```python
from build123d import *

# Parameters (mm, degrees)
F0_R     = 10
F1_DEPTH = 40
F3_D     = 10


# Not quite as in the source:
# - a feature names something its author has since deleted; it is built from what else it names


with BuildPart() as f1:
    # F0 (on Front) → F1 (new body)
    with BuildSketch(Plane.XZ):
        with BuildLine():
            ThreePointArc((-24.4948974278, 0), (-21.3326197677, -1.1270166538), (-19.5959179423, -4))
            ThreePointArc((-19.5959179423, -4), (0, -20), (19.5959179423, -4))
            ThreePointArc((19.5959179423, -4), (21.3326197677, -1.1270166538), (24.4948974278, 0))
            Line((24.4948974278, 0), (35, 0))
            ThreePointArc((35, 0), (38.5355339059, 1.4644660941), (40, 5))
            Line((40, 5), (40, 20))
            Line((40, 20), (-40, 20))
            Line((-40, 20), (-40, 5.3399834782))
            ThreePointArc((-40, 5.3399834782), (-38.6653317972, 1.5867843161), (-35.0115722683, 0))
            Line((-35.0115722683, 0), (-24.4948974278, 0))
        make_face()
        Circle(F0_R, mode=Mode.SUBTRACT)
    extrude(amount=F1_DEPTH)

    # F3 (through all)
    with Locations(Plane.XY.offset(20)):
        with Locations((-30, -10), (-29.9999981744, -30), (30, -30), (30, -10)):
            Hole(F3_D / 2)


solid = f1.part
```
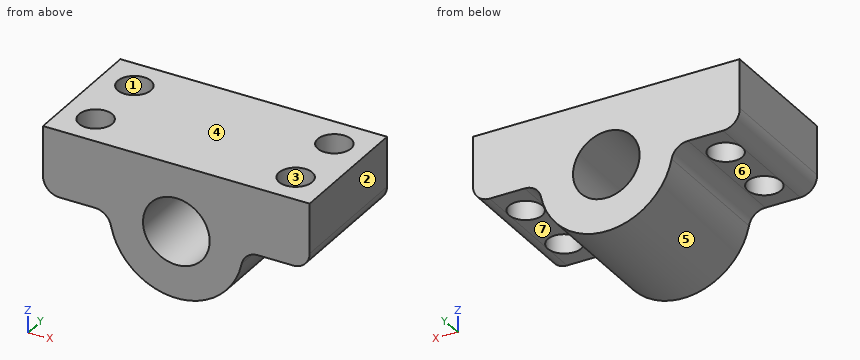
Here's how the part is built. I have some questions about the finished solid (model axes, mm). Face numbers are marked on the shaded views. A direction names the side the tool comes from. Give positions to 0.01 mm unless a question says otherwise; leave off trailing zeros. Write each loop counter-clockwise with the first axis right and the second up, starting at its lowest first coordinate (ties: lowest second). Pieces come first, ordered by that corner, then holes.
(1) Imagine slicing it at C-C, the plane z = 4. Write out the boundary of the cut face in (x, y).
Output values:
outline: (-39.91, -40) - (-9.17, -40) - (-9.17, 0) - (-39.91, 0) - close; (9.17, -40) - (39.9, -40) - (39.9, 0) - (9.17, 0) - close; hole circle Ø10 at (-30, -30); hole circle Ø10 at (-30, -10); hole circle Ø10 at (30, -30); hole circle Ø10 at (30, -10)
(2) Imagine slicing it at B-B, the plane x = -30. Write out the boundary of the cut face in (y, z).
Output values:
outline: (-40, 0) - (-35, 0) - (-35, 20) - (-40, 20) - close; (-25, 0) - (-15, 0) - (-15, 20) - (-25, 20) - close; (-5, 0) - (0, 0) - (0, 20) - (-5, 20) - close
(3) Thinking about a two-plate mould opening in X: for the marked faces 1, 2, 3 and 4, which applies, pulls with the +X half, pulls with the -X half, needs draft (parallel to the pull), parting line crosses it, or undercut?
Output values:
face 1: undercut
face 2: pulls with the +X half
face 3: undercut
face 4: needs draft
(4) Imagine slicing it at A-A, the plane y = -33. Write out the boundary of the cut face in (x, z), and give its area (3 significant figures).
Output values:
outline: (-40, 5.34) arc R5 ccw to (-35.01, 0) - (-34, 0) - (-34, 20) - (-40, 20) - close; (-26, 0) - (-24.49, 0) arc R5 cw to (-19.6, -4) arc R20 ccw to (19.6, -4) arc R5 cw to (24.49, 0) - (26, 0) - (26, 20) - (-26, 20) - close; (34, 0) - (35, 0) arc R5 ccw to (40, 5) - (40, 20) - (34, 20) - close; hole circle Ø20 at (0, 0)
area: 1,590 mm2
(5) Imagine slicing it at D-D, the plane x = 0. Write out the boundary of the cut face in (y, z), and give its area (3 significant figures).
Output values:
outline: (-40, -20) - (0, -20) - (0, -10) - (-40, -10) - close; (-40, 10) - (0, 10) - (0, 20) - (-40, 20) - close
area: 800 mm2
(6) If I drill on L1, parallel to Y at x = 30, z = 4.25; L2, parallel to X at y = -13, z = 3; L3, parallel to Y at x = -26, z = 18.5, over which ranges is the centre line in solid material (lowest first)?
Output values:
L1: y = -40 to -35, -25 to -15, -5 to 0
L2: x = -39.59 to -34, -26 to -9.54, 9.54 to 26, 34 to 39.58
L3: y = -40 to -33, -27 to -13, -7 to 0
(7) Will these pins go through, and if not, where does the flat tip stop? pin 1 (6 mm diameter, centred on x = 30, y = -30, fed in from -Z); pin 2 (10 mm diameter, centred on x = -17.5, y = -12.5, fed in from -Z); pin 3 (6 mm diameter, centred on y = -5.5, z = -4.5, fed in from +X); pin 4 (16 mm diameter, centred on x = 30, y = -10, fed in from -Z).
Output values:
pin 1: passes through
pin 2: stops at z = -15.61
pin 3: stops at x = 20.92
pin 4: stops at z = -0.67
(8) On a 3-axis mill with a long thin cutter (end or side, diameter ignored), from which of +Z, -Z, +X, -X, +Y, -Y can I reach the whole of each face in a straight line? I mean the marked faces 5, 6 and 7. Say none if no direction works.
Output values:
face 5: -Z, +Y, -Y
face 6: -Z, -X, +Y, -Y
face 7: -Z, +X, +Y, -Y
